```python
from build123d import *

# Parameters (mm, degrees)
SKETCH_1_W          = 40
SKETCH_1_H          = 70
EXTRUDE_1_DEPTH     = 3
SKETCH_2_W          = 22
SKETCH_2_H          = 61
EXTRUDE_2_DEPTH     = 3
SKETCH_3_W          = 22
SKETCH_3_H          = 7
EXTRUDE_3_DEPTH     = 12
SKETCH_4_R          = 11
EXTRUDE_4_DEPTH     = 7
SKETCH_7_R          = 1.6
CUT_EXTRUDE_2_DEPTH = 7
SKETCH_8_R          = 1.6
CUT_EXTRUDE_3_DEPTH = 7
FILLET_1_R          = 4
EXTRUDE_START       = -7
EXTRUDE_5_DEPTH     = 7
CUT_EXTRUDE_4_DEPTH = 66.76473219
CHAMFER_1_SIZE      = 2
CUT_EXTRUDE_5_DEPTH = 69.820418482


with BuildPart() as part:
    # 草图1 → 凸台-拉伸1 (new body)
    with BuildSketch(Plane.XY):
        Rectangle(SKETCH_1_W, SKETCH_1_H)
    extrude(amount=EXTRUDE_1_DEPTH)

    # 草图2 → 凸台-拉伸2 (add)
    with BuildSketch(Plane.XY.offset(3)):
        Rectangle(SKETCH_2_W, SKETCH_2_H)
    extrude(amount=-EXTRUDE_2_DEPTH)

    # 草图3 → 凸台-拉伸3 (add)
    with BuildSketch(Plane.XY.offset(3)):
        with Locations((0, -22)):
            Rectangle(SKETCH_3_W, SKETCH_3_H)
    extrude(amount=EXTRUDE_3_DEPTH)

    # 草图4 → 凸台-拉伸4 (add)
    with BuildSketch(Plane.XZ.offset(25.5)):
        with Locations((0, 15)):
            Circle(SKETCH_4_R)
    extrude(amount=-EXTRUDE_4_DEPTH)

    # 草图7 → 切除-拉伸2 (cut)
    with BuildSketch(Plane.XY.offset(3)):
        with Locations((-15, 30)):
            Circle(SKETCH_7_R)
        with Locations((15, 30)):
            Circle(SKETCH_7_R)
        with Locations((15, -30)):
            Circle(SKETCH_7_R)
        with Locations((-15, -30)):
            Circle(SKETCH_7_R)
    extrude(amount=-CUT_EXTRUDE_2_DEPTH, mode=Mode.SUBTRACT)

    # 草图8 → 切除-拉伸3 (cut)
    with BuildSketch(Plane.XY.offset(3)):
        with Locations((0, 31)):
            Circle(SKETCH_8_R)
        with Locations((0, -31)):
            Circle(SKETCH_8_R)
    extrude(amount=-CUT_EXTRUDE_3_DEPTH, mode=Mode.SUBTRACT)

    # 圆角1
    fillet_1_edges = [part.edges().sort_by_distance(p)[0] for p in [
        (20, -35, 1.5),
        (-20, -35, 1.5),
        (-20, 35, 1.5),
        (20, 35, 1.5),
    ]]
    fillet(fillet_1_edges, radius=FILLET_1_R)

    # 草图9 → 凸台-拉伸5 (add)
    with BuildSketch(Plane(origin=(0, 22, 0), x_dir=(1, 0, 0), z_dir=(0, 1, 0)).offset(EXTRUDE_START)):
        with BuildLine():
            Line((-11, -3), (-11, -15))
            ThreePointArc((-11, -15), (0, -26), (11, -15))
            Line((11, -15), (11, -3))
            Line((11, -3), (-11, -3))
        make_face()
    extrude(amount=EXTRUDE_5_DEPTH)

    # 草图10 → 切除-拉伸4 (cut, through all)
    with BuildSketch(Plane(origin=(0, 22, 0), x_dir=(1, 0, 0), z_dir=(0, 1, 0))):
        with BuildLine():
            Line((-3, -19), (3, -19))
            ThreePointArc((3, -19), (3.707106781, -18.707106781), (4, -18))
            Line((4, -18), (4, -12))
            ThreePointArc((4, -12), (3.707106781, -11.292893219), (3, -11))
            Line((3, -11), (-3, -11))
            ThreePointArc((-3, -11), (-3.707106781, -11.292893219), (-4, -12))
            Line((-4, -12), (-4, -18))
            ThreePointArc((-4, -18), (-3.707106781, -18.707106781), (-3, -19))
        make_face()
    extrude(amount=-CUT_EXTRUDE_4_DEPTH, mode=Mode.SUBTRACT)

    # 倒角1
    chamfer_1_edges = [part.edges().sort_by_distance(p)[0] for p in [
        (-11, 18.5, 3),
        (11, 18.5, 3),
        (11, -22, 3),
        (-11, -22, 3),
    ]]
    chamfer(chamfer_1_edges, length=CHAMFER_1_SIZE)

    # 草图11 → 切除-拉伸5 (cut, through all)
    with BuildSketch(Plane.XZ.offset(25.5)):
        with BuildLine():
            Line((-4.1, 18), (-4.1, 12))
            ThreePointArc((-4.1, 12), (-3.777817459, 11.222182541), (-3, 10.9))
            Line((-3, 10.9), (3, 10.9))
            ThreePointArc((3, 10.9), (3.777817459, 11.222182541), (4.1, 12))
            Line((4.1, 12), (4.1, 18))
            ThreePointArc((4.1, 18), (3.777817459, 18.777817459), (3, 19.1))
            Line((3, 19.1), (-3, 19.1))
            ThreePointArc((-3, 19.1), (-3.777817459, 18.777817459), (-4.1, 18))
        make_face()
    extrude(amount=-CUT_EXTRUDE_5_DEPTH, mode=Mode.SUBTRACT)


solid = part.part
```
The model under review builds one solid part; all positions refer to its coordinate system, in mm. A direction names the side the tool comes from. Coordinates: 2 decimals unless noted, no trailing zeros. Write each loop counter-clockwise with the first axis right and the second up, starting at its lowest first coordinate (ties: lowest second). Pieces come first, ordered by that corner, then holes. Notation, with made-up numbers: (4.25, -37.5) - (47.25, -37.5) arc R26 cw to (47.25, -20.5) - close; hole circle Ø11 at (79.5, 26). An arc over 180 degrees is marked (long way). Write item = value, one per line.
(1) For line 1 (Y direction, x = -15, z = 2.1); line 2 (Y direction, x = 0, z = 1.9); line 3 (Y direction, x = 8.5, z = 3.5), list the stretches that pass through material, from the lowest coordinate up. Write a range as [from, to].
Result sheet:
line_1 = [-35, -31.6], [-28.4, 28.4], [31.6, 35]
line_2 = [-35, -32.6], [-29.4, 29.4], [32.6, 35]
line_3 = [-25.5, -18.5], [15, 22]
(2) Machinability: for faces 1 (the face through (0, 15, 9)), 2 (the face through (-11, -22, 10)), 3 (the face through (4.1, -22, 15)), which of the approach directions +Z, -Z, +X, -X, +Y, -Y give a long, thin tool a straight path to every point of the face, cutting with its end or side? Answer none if there is none.
Result sheet:
face_1 = +Z, +X, -X
face_2 = +Z, -X, +Y, -Y
face_3 = +Y, -Y
(3) Consider section B-B, the plane z = 3.75. Give the boundary of the cut face in (x, y), then the cut area to 3 significant figures.
Result sheet:
outline = (-12.25, -25.5) - (12.25, -25.5) - (12.25, -18.5) - (-12.25, -18.5) - close; (-12.25, 15) - (12.25, 15) - (12.25, 22) - (-12.25, 22) - close
area = 343 mm^2
(4) Consider section C-C, the plane y = -22. Give the boundary of the cut face in (x, z).
Result sheet:
outline = (-20, 0) - (20, 0) - (20, 3) - (13, 3) - (11, 5) - (11, 15) arc R11 ccw to (-11, 15) - (-11, 5) - (-13, 3) - (-20, 3) - close; hole (-4.1, 12) arc R1.1 ccw to (-3, 10.9) - (3, 10.9) arc R1.1 ccw to (4.1, 12) - (4.1, 18) arc R1.1 ccw to (3, 19.1) - (-3, 19.1) arc R1.1 ccw to (-4.1, 18) - close
(5) For P1, Ø5, axis at y = -22.5, z = 16, coming from the +X side; P2, Ø7.5, axis at y = -23.5, z = 7.5, coming from the +X side; P3, Ø12, axis at x = -3, y = 5.5, coming from the +Z side, all flat-tipped, find the tip position at first contact; note any pin that passes through.
Result sheet:
P1 = 11
P2 = 12.25
P3 = 3
(6) Mouldability with a two-part tool opening along Z and no side actions: class faces 4 (the face through (0, -22, 26)), 5 (the face through (0, -35, 1)), 6 (the face through (0, -22, 10.9)) as pulls with the +Z half, pulls with the -Z half, needs draft (parallel to the pull), parting line crosses it, or undercut.
Result sheet:
face_4 = pulls with the +Z half
face_5 = needs draft
face_6 = undercut
(7) Consider section D-D, the plane x = 0. Give the boundary of the cut face in (y, z).
Result sheet:
outline = (-35, 0) - (-32.6, 0) - (-32.6, 3) - (-35, 3) - close; (-29.4, 0) - (29.4, 0) - (29.4, 3) - (22, 3) - (22, 10.9) - (15, 10.9) - (15, 3) - (-18.5, 3) - (-18.5, 10.9) - (-25.5, 10.9) - (-25.5, 3) - (-29.4, 3) - close; (-25.5, 19.1) - (-18.5, 19.1) - (-18.5, 26) - (-25.5, 26) - close; (15, 19.1) - (22, 19.1) - (22, 26) - (15, 26) - close; (32.6, 0) - (35, 0) - (35, 3) - (32.6, 3) - close
(8) Consider section A-A, the plane x = -15. Give the boundary of the cut face in (y, z).
Result sheet:
outline = (-35, 0) - (-31.6, 0) - (-31.6, 3) - (-35, 3) - close; (-28.4, 0) - (28.4, 0) - (28.4, 3) - (-28.4, 3) - close; (31.6, 0) - (35, 0) - (35, 3) - (31.6, 3) - close
